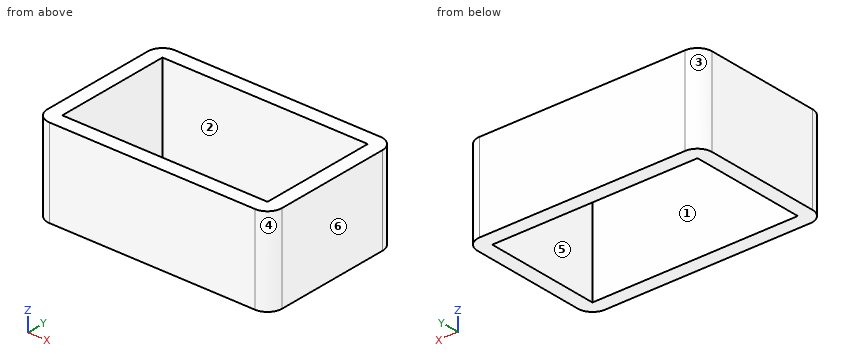
from build123d import *

# Parameters (mm, degrees)
F0_W     = 80
F0_H     = 50
F1_DEPTH = 30
F2_W     = 70
F2_H     = 40
F3_DEPTH = 30.001
F4_R     = 5


with BuildPart() as f1:
    # F0 (on Top) → F1 (new body)
    with BuildSketch(Plane.XY):
        with Locations((40, 25)):
            Rectangle(F0_W, F0_H)
    extrude(amount=F1_DEPTH)

    # F2 (on face) → F3 (cut, through all)
    with BuildSketch(Plane.XY.offset(30)):
        with Locations((40, 25)):
            Rectangle(F2_W, F2_H)
    extrude(amount=-F3_DEPTH, mode=Mode.SUBTRACT)

    # F4
    f4_edges = [f1.edges().sort_by_distance(p)[0] for p in [
        (0, 0, 15),
        (80, 0, 15),
        (0, 50, 15),
        (80, 50, 15),
    ]]
    fillet(f4_edges, radius=F4_R)


solid = f1.part
Verification items for the finished model (mm, model axes). Face numbers are marked on the shaded views. A direction names the side the tool comes from. Give positions to 0.01 mm unless a question says otherwise; leave off trailing zeros. Loops run counter-clockwise (first coordinate to the right, second up) from the corner with the lowest first, then second, coordinate; pieces in that order, holes last.
1) Draft check along Y on the marked faces 1, 2, 3 and 4. Enter one of: pulls with the +Y half, pulls with the -Y half, needs draft (parallel to the pull), parting line crosses it, or undercut.
2) Thickness scan on line 1 along X through (y, z) = (29, 12.5); line 2 along Y through (x, z) = (42.5, 18). Record the ranges inside material, lowest first.
3) Sectioned sample at B-B, the plane y = 43. Enter the section's corners in (x, z).
4) Sectioned sample at A-A, the plane x = 21. Enter the section's corners in (y, z), then the cut area to 3 significant figures.
5) Depth check by flat-ended pin: pin 1 Ø12 at (x, y) = (60.5, 15.5) entering from -Z. Enter the tip coordinate at first touch or a pass-through.
6) Set-up check for the marked faces 5 and 6: record each of +Z, -Z, +X, -X, +Y, -Y from which the full face is reachable in a straight line by a thin tool's end or side.
7) Sectioned sample at C-C, the plane z = 16. Enter the section's corners in (x, y).
Answers:
1. face 1: undercut
1. face 2: undercut
1. face 3: pulls with the +Y half
1. face 4: pulls with the -Y half
2. line 1: x = 0 to 5, 75 to 80
2. line 2: y = 0 to 5, 45 to 50
3. outline: (0, 0) - (5, 0) - (5, 30) - (0, 30) - close; (75, 0) - (80, 0) - (80, 30) - (75, 30) - close
4. outline: (0, 0) - (5, 0) - (5, 30) - (0, 30) - close; (45, 0) - (50, 0) - (50, 30) - (45, 30) - close
4. area: 300 mm2
5. pin 1: passes through
6. face 5: +Z, -Z
6. face 6: +Z, -Z, +X, +Y, -Y
7. outline: (0, 5) arc R5 ccw to (5, 0) - (75, 0) arc R5 ccw to (80, 5) - (80, 45) arc R5 ccw to (75, 50) - (5, 50) arc R5 ccw to (0, 45) - close; hole (5, 5) - (75, 5) - (75, 45) - (5, 45) - close
